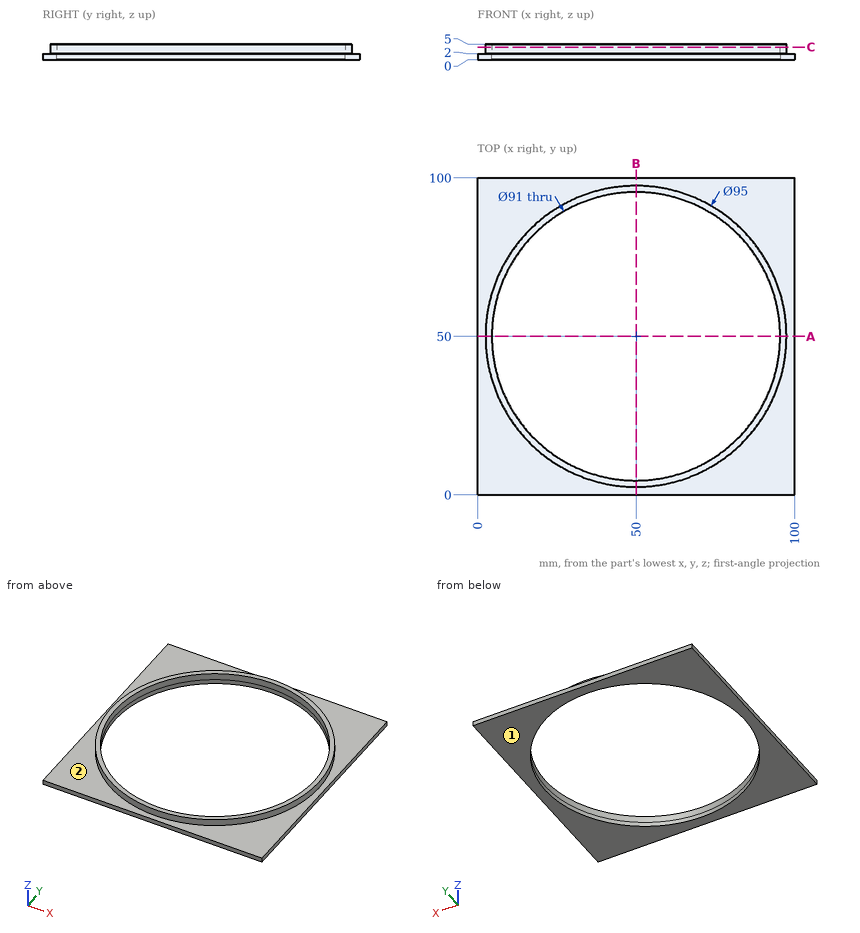
Could you check a few things on this drawing? It's one solid part, dimensions in mm from its lowest x, y, z. A direction names the side the tool comes from. Coordinates: 2 decimals unless noted, no trailing zeros. Order: outer loops, then holes, each group sorted by start corner. A loop starts at its lowest first (then second) coordinate and runs counter-clockwise, first axis right, second up. Notation, with made-up numbers: M 30,1.5 L 66,1.5 A21 cw 66,28.5 Z; hole C 14,64.25 d5. An arc over 180 degrees is marked long. Use one line per item in the form item = value. Start each with the question number.
1. On a 3-axis mill with a long thin cutter (end or side, diameter ignored), from which of +Z, -Z, +X, -X, +Y, -Y can I reach the whole of each face in a straight line? I mean the marked faces 1 and 2. Say none if no direction works.
2. For pin 1 (1 mm diameter, centred on x = 29.5, z = 3.5, fed in from -Y); pin 2 (10 mm diameter, centred on x = 39.5, y = 88.5, fed in from -Z), each with a flat end and sliding along its axis, tell me the tip position at first contact or that it passes through.
3. Suppose I cut it at A-A on y = 50. Write out the boundary of the cut face in (x, z).
4. Suppose I cut it at C-C on z = 4. Write out the boundary of the cut face in (x, y), then the cut area to 3 significant figures.
5. Please list where these lines run through material, in increasing order: line 1 (Y direction, x = 49, z = 3.6); line 2 (Y direction, x = 50, z = 1.2); line 3 (Z direction, x = 78.5, y = 90).
Geometry says:
q1.face_1 = -Z, +X, -X, +Y, -Y
q1.face_2 = +Z
q2.pin_1 = 6.92
q2.pin_2 = through
q3.outline = M 0,0 L 4.5,0 L 4.5,5 L 2.5,5 L 2.5,2 L 0,2 Z; M 95.5,0 L 100,0 L 100,2 L 97.5,2 L 97.5,5 L 95.5,5 Z
q4.outline = C 50,50 d95; hole C 50,50 d91
q4.area = 584 mm^2
q5.line_1 = 2.51 to 4.51, 95.49 to 97.49
q5.line_2 = 0 to 4.5, 95.5 to 100
q5.line_3 = 0 to 2
